Autodesk Inventor part; units mm, degrees
ref_plane "YZ Plane" through (0, 0, 0) normal (1, 0, 0) x (0, 1, 0)
ref_plane "XZ Plane" through (0, 0, 0) normal (0, 1, 0) x (-1, 0, 0)
ref_plane "XY Plane" through (0, 0, 0) normal (0, 0, 1) x (1, 0, 0)
sketch "Sketch1" plane through (0, 0, 0) normal (0, 0, 1) x (1, 0, 0)
  line L0 (0, 0) -> (76.2, 0)
  line L1 (76.2, 0) -> (76.2, 38.1)
  line L2 (57.15, 50.8) -> (31.75, 50.8)
  line L3 (57.15, 50.8) -> (76.2, 38.1)
  line L4 (0, 0) -> (0, 6.35)
  line L5 (0, 6.35) -> (19.05, 6.35)
  line L6 (19.05, 6.35) -> (19.05, 19.05)
  line L7 (19.05, 19.05) -> (0, 19.05)
  line L8 (0, 19.05) -> (0, 31.75)
  line L9 (0, 31.75) -> (31.75, 50.8)
  line L10 (76.2, 0) -> (50.8, 0)
  circle A0 centre (50.8, 25.4) radius 12.7
  dimension "d0" = 76.2
  dimension "d1" = 38.1
  dimension "d4" = 25.4
  dimension "d5" = 6.35
  dimension "d6" = 19.05
  dimension "d7" = 12.7
  dimension "d8" = 19.05
  dimension "d9" = 12.7
  dimension "d10" = 25.4
  dimension "d12" = 25.4
extrude "Extrusion1" add sketch "Sketch1" along normal blind 12.7
properties part number "Assignment 1.1 - Inclined Support"
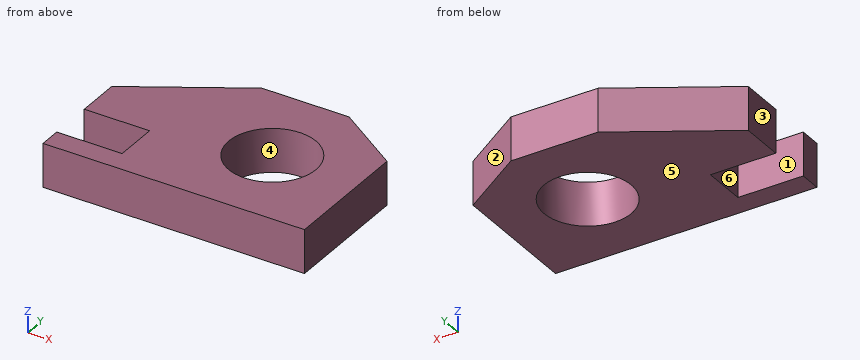
Source: CAD feature listing. Evaluate the final solid. Frame: model axes, mm. Face numbers are marked on the shaded views. A direction names the side the tool comes from. Round coordinates to 2 decimals unless told otherwise and drop trailing zeros. Write each loop counter-clockwise with the first axis right and the second up, starting at its lowest first coordinate (ties: lowest second). Pieces come first, ordered by that corner, then holes. Notation, with made-up numbers: M 67.5,46 L 109.5,46 A13 cw 109.5,57 Z; hole C 57.5,-31 d1. An arc over 180 degrees is marked long. One line per item, written item: value. Start each with the question number.
Item 1: Set-up query: the marked faces 5 and 6. Return all of +Z, -Z, +X, -X, +Y, -Y with unobstructed straight access to the full face (end or side cutting, diameter ignored); none if empty.
Item 2: Section query C-C (x = 60.5). Return the cut outline in (y, z), plus the area to 3 significant figures.
Item 3: Section query A-A (z = 1). Return the cut outline in (x, y), plus the area to 3 significant figures.
Item 4: Section query B-B (y = 25.4). Return the cut outline in (x, z), plus the area to 3 significant figures.
Item 5: Pin query (flat end, axial travel): pin 1 (3 mm diameter, centred on x = 62.5, y = 24.5, fed in from +Z); pin 2 (1 mm diameter, centred on y = 41, z = 11.5, fed in from -X); pin 3 (4 mm diameter, centred on x = 12.5, z = 5.5, fed in from +Y); pin 4 (3 mm diameter, centred on y = 40, z = 4.5, fed in from -X). Return the tip coordinate at first contact, or that it passes through.
Item 6: Section query D-D (y = 47.5). Return the cut outline in (x, z), plus the area to 3 significant figures.
Item 7: Mould query, pull axis X, two halves, no side actions, for the marked faces 1, 2, 3 and 4. Classes: pulls with the +X half, pulls with the -X half, needs draft (parallel to the pull), parting line crosses it, or undercut.
Item 8: Ray query, L1, parallel to X at y = 25, z = 5.25; L2, parallel to Y at x = 50.8, z = 6.25; L3, parallel to X at y = 7.5, z = 7.5. Return the intervals inside material, ascending. Write a range as from..to.
Result set:
1. face 5: -Z, +X, -X, +Y, -Y
1. face 6: +Z, -Z, -X
2. outline: M 0,0 L 17.2,0 L 17.2,12.7 L 0,12.7 Z; M 33.6,0 L 48.57,0 L 48.57,12.7 L 33.6,12.7 Z
2. area: 409 mm²
3. outline: M 0,0 L 76.2,0 L 76.2,38.1 L 57.15,50.8 L 31.75,50.8 L 0,31.75 L 0,19.05 L 19.05,19.05 L 19.05,6.35 L 0,6.35 Z; hole C 50.8,25.4 d25.4
3. area: 2,700 mm²
4. outline: M 0,0 L 38.1,0 L 38.1,12.7 L 0,12.7 Z; M 63.5,0 L 76.2,0 L 76.2,12.7 L 63.5,12.7 Z
4. area: 645 mm²
5. pin 1: stops at z = 12.7
5. pin 2: stops at x = 14.58
5. pin 3: stops at y = 40.45
5. pin 4: stops at x = 11.25
6. outline: M 26.25,0 L 62.1,0 L 62.1,12.7 L 26.25,12.7 Z
6. area: 455 mm²
7. face 1: needs draft
7. face 2: pulls with the +X half
7. face 3: pulls with the -X half
7. face 4: undercut
8. L1: x = 0..38.11, 63.49..76.2
8. L2: y = 0..12.7, 38.1..50.8
8. L3: x = 19.05..76.2
